Work out the finished part from the listing and answer in its coordinate system (mm). A direction names the side the tool comes from. Coordinates: 2 decimals unless noted, no trailing zeros. Order: outer loops, then holes, each group sorted by start corner. A loop starts at its lowest first (then second) coordinate and runs counter-clockwise, first axis right, second up. Notation, with made-up numbers: M 57,17 L 111,17 A21 ccw 111,21 Z; hole C 6.25,31.5 d4. An arc over 180 degrees is marked long. Use a Markdown table: item, result.
from build123d import *

# Parameters (mm, degrees)
TORUS_R           = 4
CYLINDER003_R     = 18
CYLINDER003_DEPTH = 2
BOX_W             = 7
BOX_H             = 41
BOX_DEPTH         = 10
CYLINDER002_R     = 18
CYLINDER002_DEPTH = 10
CYLINDER001_R     = 75
CYLINDER001_DEPTH = 4
CYLINDER_R        = 61
CYLINDER_DEPTH    = 10


with BuildPart() as torus:
    # Torus → Torus (revolve)
    with BuildSketch(Plane.XZ):
        with Locations((40, 0)):
            Circle(TORUS_R)
    revolve(axis=Axis((0, 0, 0), (0, 0, 1)))


with BuildPart() as cylinder003:
    # Cylinder003 → Cylinder003 (new body)
    with BuildSketch(Plane.XY.offset(8)):
        Circle(CYLINDER003_R)
    extrude(amount=CYLINDER003_DEPTH)


with BuildPart() as box:
    # Box → Box (new body)
    with BuildSketch(Plane(origin=(-3, -20, 0), x_dir=(1, 0, 0), z_dir=(0, 0, 1))):
        with Locations((3.5, 20.5)):
            Rectangle(BOX_W, BOX_H)
    extrude(amount=BOX_DEPTH)


with BuildPart() as cylinder002:
    # Cylinder002 → Cylinder002 (new body)
    with BuildSketch(Plane.XY):
        Circle(CYLINDER002_R)
    extrude(amount=CYLINDER002_DEPTH)


with BuildPart() as cylinder001:
    # Cylinder001 → Cylinder001 (new body)
    with BuildSketch(Plane.XY):
        Circle(CYLINDER001_R)
    extrude(amount=CYLINDER001_DEPTH)


with BuildPart() as cut001:
    # Cylinder → Cylinder (new body)
    with BuildSketch(Plane.XY):
        Circle(CYLINDER_R)
    extrude(amount=CYLINDER_DEPTH)

    # Fusion: union Cylinder001
    add(cylinder001.part)

    # Cut: cut Cylinder002
    add(cylinder002.part, mode=Mode.SUBTRACT)

    # Fusion001: union Box
    add(box.part)

    # Fusion002: union Cylinder003
    add(cylinder003.part)

    # Cut001: cut Torus
    add(torus.part, mode=Mode.SUBTRACT)


solid = cut001.part
1. Section A-A on z = 2 is taken. Determine the outline of the cut face in (x, y).
Answers below:
| item | result |
|---|---|
| outline | C 0,0 d150; C 0,0 d73.07; hole C 0,0 d86.93; hole M -3,-17.75 L -3,17.75 A18 ccw Z; hole M 4,-17.55 A18 ccw 4,17.55 Z |
2. Section D-D on y = 53.5 is taken. Determine the outline of the cut face in (x, z).
Answers below:
| item | result |
|---|---|
| outline | M -52.56,0 L 52.56,0 L 52.56,4 L 29.3,4 L 29.3,10 L -29.3,10 L -29.3,4 L -52.56,4 Z |
3. Find the intervals of material crossed by probe 1 along X at (y, z) = (-25.5, 3.25); probe 2 along Y at (x, z) = (-14, 1.5); probe 3 along X at (y, z) = (27.5, 1.25), in increasing order.
Answers below:
| item | result |
|---|---|
| probe 1 | -70.53 to -33.79, -27.72 to 27.72, 33.79 to 70.53 |
| probe 2 | -73.68 to -41.41, -33.48 to -11.31, 11.31 to 33.48, 41.41 to 73.68 |
| probe 3 | -69.78 to -34.09, -23.54 to 23.54, 34.09 to 69.78 |
4. For faces 4 (the face through (-9.764, 74.362, 1.972)), 5 (the face through (9, 0, 8)), 6 (the face through (11, -61, 4)), determine the directions among +Z, -Z, +X, -X, +Y, -Y from which every point of the face is accessible in a straight line to the end or side of a thin tool.
Answers below:
| item | result |
|---|---|
| face 4 | +Z, -Z |
| face 5 | -Z |
| face 6 | +Z |
5. Section B-B on y = 0 is taken. Determine the outline of the cut face in (x, z), then the cut area to 3 significant figures.
Answers below:
| item | result |
|---|---|
| outline | M -75,0 L -44,0 A4 cw -36,0 L -18,0 L -18,8 L -3,8 L -3,0 L 4,0 L 4,8 L 18,8 L 18,0 L 36,0 A4 cw 44,0 L 75,0 L 75,4 L 61,4 L 61,10 L -61,10 L -61,4 L -75,4 Z |
| area | 1,050 mm² |
6. For a pull along X with two mould halves and no side action, classify faces 1 (the face through (-1, 1, 0)), 2 (the face through (-48.408, -37.118, 6.958)), 3 (the face through (-9, 0, 8)) as +X half, -X half, draft (parallel to the pull), parting line (faces both ways), or undercut.
Answers below:
| item | result |
|---|---|
| face 1 | draft |
| face 2 | parting line |
| face 3 | undercut |
7. Flat-ended cylindrical pins translate along their axes: P1, Ø4, axis at y = -2, z = 2, coming from the -X side; P2, Ø3, axis at x = 12.5, y = -36.5, coming from the -Z side; P3, Ø6, axis at x = -23.5, z = 8.5, coming from the -Y side; P4, Ø6, axis at x = -24, z = 1.5, coming from the -Y side. Find the tip coordinate at first contact, or state that the pin passes through.
Answers below:
| item | result |
|---|---|
| P1 | x = -75 |
| P2 | z = 2.73 |
| P3 | y = -57.45 |
| P4 | y = -72 |
8. Section C-C on x = 0 is taken. Determine the outline of the cut face in (y, z).
Answers below:
| item | result |
|---|---|
| outline | M -75,0 L -44,0 A4 cw -36,0 L 36,0 A4 cw 44,0 L 75,0 L 75,4 L 61,4 L 61,10 L -61,10 L -61,4 L -75,4 Z |
